from build123d import *

# Parameters (mm, degrees)
SKETCH_1_R          = 5
EXTRUDE_1_DEPTH     = 150
SKETCH_2_R          = 9
EXTRUDE_2_DEPTH     = 5
CUT_EXTRUDE_1_REACH = 161.568
SKETCH_3_R          = 2.5


with BuildPart() as part:
    # 草图1 → 凸台-拉伸1 (new, symmetric)
    with BuildSketch(Plane(origin=(0, 0, 0), x_dir=(1, 0, 0), z_dir=(0, 1, 0))):
        with Locations(Location((0, 0, 0), (0, 0, 270))):
            Circle(SKETCH_1_R)
    extrude(amount=EXTRUDE_1_DEPTH, both=True)

    # 草图2 → 凸台-拉伸2 (add, symmetric)
    with BuildSketch(Plane.XY):
        with Locations((0, 150)):
            Circle(SKETCH_2_R)
        with Locations((0, -150)):
            Circle(SKETCH_2_R)
    extrude(amount=EXTRUDE_2_DEPTH, both=True)

    # 草图3 → 切除-拉伸1 (cut, up to next)
    with BuildSketch(Plane.XY.offset(5), mode=Mode.PRIVATE) as cut_extrude_1_sk1:
        with Locations((0, 150)):
            Circle(SKETCH_3_R)
    cut_extrude_1_tool1 = extrude(cut_extrude_1_sk1.sketch, amount=-CUT_EXTRUDE_1_REACH, mode=Mode.PRIVATE) & part.part
    # 草图3 → 切除-拉伸1 (cut, up to next)
    with BuildSketch(Plane.XY.offset(5), mode=Mode.PRIVATE) as cut_extrude_1_sk2:
        with Locations((0, -150)):
            Circle(SKETCH_3_R)
    cut_extrude_1_tool2 = extrude(cut_extrude_1_sk2.sketch, amount=-CUT_EXTRUDE_1_REACH, mode=Mode.PRIVATE) & part.part
    add(cut_extrude_1_tool1.solids().sort_by_distance((0, 150, 5))[0], mode=Mode.SUBTRACT)
    add(cut_extrude_1_tool2.solids().sort_by_distance((0, -150, 5))[0], mode=Mode.SUBTRACT)


solid = part.part
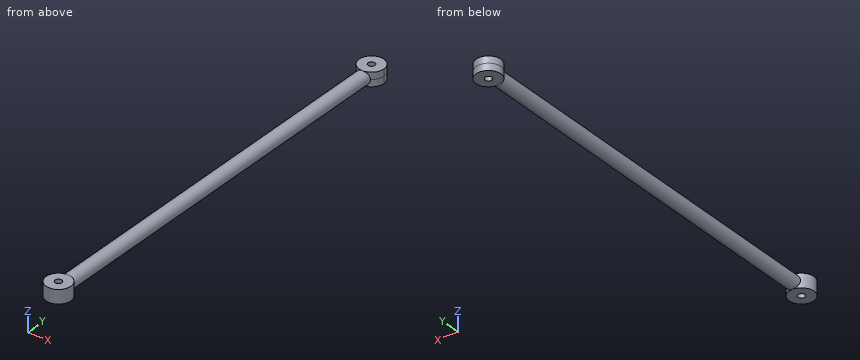
Read the model definition and answer for the solid it produces. Units are mm, in the model's axes. Give positions to 0.01 mm unless a question says otherwise; leave off trailing zeros. Write each loop counter-clockwise with the first axis right and the second up, starting at its lowest first coordinate (ties: lowest second). Pieces come first, ordered by that corner, then holes. Notation, with made-up numbers: M -9,-18.5 L 18,-18.5 A28 cw 18,17.5 Z; hole C -5,88.25 d3. An arc over 180 degrees is marked long. One line per item, written item: value. Start each with the question number.
(1) Find the intervals of material crossed by line 1 (Y direction, x = -0.5, z = -3); line 2 (Y direction, x = 0, z = -1); line 3 (X direction, y = 150, z = -0.25), in increasing order.
(2) Find section A-A (z = 3). Determine the outline of the cut face in (x, y).
(3) Flat-ended cylindrical pins translate along their axes: pin 1 Ø4 at (x, y) = (0, 150) entering from -Z; pin 2 Ø1 at (y, z) = (91, 2.5) entering from +X; pin 3 Ø3 at (x, y) = (-2.5, -11) entering from +Z; pin 4 Ø6 at (y, z) = (106, 2) entering from -X. Find the tip coordinate at first contact, or state that the pin passes through.
(4) Find section B-B (y = -39.5). Determine the outline of the cut face in (x, z).
Results below:
1. line 1: y = -158.99 to -152.45, -147.55 to 147.55, 152.45 to 158.99
1. line 2: y = -159 to -152.5, -147.5 to 147.5, 152.5 to 159
1. line 3: x = -9 to -2.5, 2.5 to 9
2. outline: M -4,-141.94 A9 ccw long 4,-141.94 L 4,141.94 A9 ccw long -4,141.94 Z; hole C 0,-150 d5; hole C 0,150 d5
3. pin 1: passes through
3. pin 2: stops at x = 4.58
3. pin 3: stops at z = 4.9
3. pin 4: stops at x = -5
4. outline: C 0,0 d10
